from build123d import *

# Parameters (mm, degrees)
SKETCH1_W            = 152.4
SKETCH1_H            = 222.25
SKETCH1_R            = 2.54
BOSS_EXTRUDE1_DEPTH  = 3.175
FILLET1_R            = 6.35
EDGE_FLANGE1_DEPTH   = 152.4
EDGE_FLANGE1_2_DEPTH = 152.4
FILLET2_R            = 6.35


# Read off the part's stored shape, not the designer's step: Edge-Flange1
with BuildPart() as part:
    # Sketch1 → Boss-Extrude1 (new body)
    with BuildSketch(Plane.XY):
        with Locations((76.2, 111.125)):
            Rectangle(SKETCH1_W, SKETCH1_H)
        with Locations((12.7, 44.45)):
            Circle(SKETCH1_R, mode=Mode.SUBTRACT)
        with Locations((38.1, 44.45)):
            Circle(SKETCH1_R, mode=Mode.SUBTRACT)
        with Locations((63.5, 44.45)):
            Circle(SKETCH1_R, mode=Mode.SUBTRACT)
        with Locations((88.9, 44.45)):
            Circle(SKETCH1_R, mode=Mode.SUBTRACT)
        with Locations((114.3, 44.45)):
            Circle(SKETCH1_R, mode=Mode.SUBTRACT)
        with Locations((139.7, 44.45)):
            Circle(SKETCH1_R, mode=Mode.SUBTRACT)
    extrude(amount=BOSS_EXTRUDE1_DEPTH)

    # Fillet1
    fillet1_edges = [part.edges().sort_by_distance(p)[0] for p in [
        (0, 222.25, 1.5875),
        (152.4, 222.25, 1.5875),
    ]]
    fillet(fillet1_edges, radius=FILLET1_R)

    # Edge-Flange1 outline → Edge-Flange1 (cut)
    with BuildSketch(Plane.YZ):
        with BuildLine():
            ThreePointArc((19.158982919, 0), (18.010706008, 0.050134853), (16.871168178, 0.200157854))
            Line((16.871168178, 0.200157854), (0, 3.175))
            Line((0, 3.175), (0, 0))
            Line((0, 0), (19.158982919, 0))
        make_face()
    extrude(amount=EDGE_FLANGE1_DEPTH, mode=Mode.SUBTRACT)

    # Edge-Flange1 2 outline → Edge-Flange1 2 (add)
    with BuildSketch(Plane.YZ):
        with BuildLine():
            Line((-57.036031002, 13.231991138), (0, 3.175))
            Line((0, 3.175), (19.158982919, 3.175))
            ThreePointArc((19.158982919, 3.175), (18.287425492, 3.213053019), (17.422501143, 3.32692247))
            Line((17.422501143, 3.32692247), (-56.484698038, 16.358755754))
            Line((-56.484698038, 16.358755754), (-57.036031002, 13.231991138))
        make_face()
    extrude(amount=EDGE_FLANGE1_2_DEPTH)

    # Fillet2
    fillet2_edges = [part.edges().sort_by_distance(p)[0] for p in [
        (0, -56.76036452, 14.795373446),
        (152.4, -56.76036452, 14.795373446),
    ]]
    fillet(fillet2_edges, radius=FILLET2_R)


solid = part.part
Can you work these out from the model? Positions are in its coordinate system, mm. A direction names the side the tool comes from. Round coordinates to 2 decimals unless told otherwise and drop trailing zeros. Write each loop counter-clockwise with the first axis right and the second up, starting at its lowest first coordinate (ties: lowest second). Pieces come first, ordered by that corner, then holes. Notation, with made-up numbers: (42, -17) -> (78, -17) arc R31 ccw to (78, 14) -> close; hole circle Ø9 at (-8.5, 3.25). An arc over 180 degrees is marked (long way). Use one line per item in the form item = value. Start each with the question number.
Q1. Imagine slicing it at B-B (y = 149.5). Please give me the cut outline in (x, z) (3 decimals).
Q2. I'm going to push flat-ended pins straight in: P1, Ø4.5, axis at x = 88.9, y = 44.45, coming from the -Z side; P2, Ø6, axis at x = 38.1, y = 44.45, coming from the -Z side; P3, Ø6.5, axis at x = 63.5, y = 44.45, coming from the +Z side (3 decimals); P4, Ø6, axis at x = 74.5, y = -22, coming from the +Z side. Where does each tip first touch, or does it pass through?
Q3. If I drill on probe 1 along Z at (x, y) = (83, 92) (3 decimals), over which ranges is the centre line in solid material (lowest first)? Write a range as [from, to].
Q4. Which directions (+Z, -Z, +X, -X, +Y, -Y) give clear straight access to the entire face, cutting with the end or side of a thin tool? Please do faces 1 (the face through (75, 122, 3.175)), 2 (the face through (111.762, 44.562, 1.565)).
Q5. We'd pull the mould along Y, two halves only. Please class faces 3 (the face through (87.03, 46.17, 1.57)), 4 (the face through (75, 122, 0)), 5 (the face through (1.81, 220.34, 1.61)): +Y half, -Y half, draft (parallel to the pull), parting line (faces both ways), or undercut.
Worked out:
q1.outline = (0, 0) -> (152.4, 0) -> (152.4, 3.175) -> (0, 3.175) -> close
q2.P1 = through
q2.P2 = 0
q2.P3 = 3.175
q2.P4 = 10.81
q3.probe_1 = [0, 3.175]
q4.face_1 = +Z, +X, -X, +Y
q4.face_2 = +Z, -Z
q5.face_3 = undercut
q5.face_4 = draft
q5.face_5 = +Y half
